```python
from build123d import *

# Parameters (mm, degrees)
F0_R     = 12
F1_DEPTH = 2
F3_DEPTH = 25


with BuildPart() as f1:
    # F0 (on Top) → F1 (new body)
    with BuildSketch(Plane.XY):
        Circle(F0_R)
    extrude(amount=F1_DEPTH)

    # F2 (on face) → F3 (cut)
    with BuildSketch(Plane.XY.offset(2)):
        Polygon((-3.2808869146, 6.2673611111), (-3.2808869146, 7.8645833333), (-5.1267361111, 7.8645833333), (-5.1267361111, -8), (-3.2808869146, -8), (-3.2808869146, -6.4270833333), (-3.2829861111, -6.4270833333), (-3.2829861111, -0.4895833333), (-3.2808869146, -0.4895833333), (-3.2808869146, 1.0729166667), (-3.2829861111, 1.0729166667), (-3.2829861111, 6.2673611111), align=None)
        with BuildLine():
            Line((-0.6440972222, 7.8645833333), (-1.7808869146, 7.8645833333))
            Line((-1.7808869146, 7.8645833333), (-1.7808869146, 6.2673611111))
            Line((-1.7808869146, 6.2673611111), (-0.5677083333, 6.2673611111))
            add(Edge.make_bspline(
                [(2.4704861111, 5.6770833333), (1.515625, 6.2673611111), (-0.5677083333, 6.2673611111)],
                knots=[0, 0, 0, 1, 1, 1], degree=2))
            add(Edge.make_bspline(
                [(3.4253472222, 3.75), (3.4253472222, 5.0868055556), (2.4704861111, 5.6770833333)],
                knots=[0, 0, 0, 1, 1, 1], degree=2))
            add(Edge.make_bspline(
                [(2.5677083333, 1.6857638889), (3.4253472222, 2.2986111111), (3.4253472222, 3.75)],
                knots=[0, 0, 0, 1, 1, 1], degree=2))
            add(Edge.make_bspline(
                [(-0.2447916667, 1.0729166667), (1.7100694444, 1.0729166667), (2.5677083333, 1.6857638889)],
                knots=[0, 0, 0, 1, 1, 1], degree=2))
            Line((-0.2447916667, 1.0729166667), (-1.7808869146, 1.0729166667))
            Line((-1.7808869146, 1.0729166667), (-1.7808869146, -0.4895833333))
            Line((-1.7808869146, -0.4895833333), (-0.1232638889, -0.4895833333))
            add(Edge.make_bspline(
                [(2.8975694444, -1.1840277778), (1.9045138889, -0.4895833333), (-0.1232638889, -0.4895833333)],
                knots=[0, 0, 0, 1, 1, 1], degree=2))
            add(Edge.make_bspline(
                [(3.890625, -3.3541666667), (3.890625, -1.8784722222), (2.8975694444, -1.1840277778)],
                knots=[0, 0, 0, 1, 1, 1], degree=2))
            add(Edge.make_bspline(
                [(2.9201388889, -5.6840277778), (3.890625, -4.9409722222), (3.890625, -3.3541666667)],
                knots=[0, 0, 0, 1, 1, 1], degree=2))
            add(Edge.make_bspline(
                [(0.0295138889, -6.4270833333), (1.9496527778, -6.4270833333), (2.9201388889, -5.6840277778)],
                knots=[0, 0, 0, 1, 1, 1], degree=2))
            Line((0.0295138889, -6.4270833333), (-1.7808869146, -6.4270833333))
            Line((-1.7808869146, -6.4270833333), (-1.7808869146, -8))
            Line((-1.7808869146, -8), (0.4079861111, -8))
            add(Edge.make_bspline(
                [(4.4288194444, -6.8055555556), (2.9913194444, -8), (0.4079861111, -8)],
                knots=[0, 0, 0, 1, 1, 1], degree=2))
            add(Edge.make_bspline(
                [(5.8663194444, -3.4861111111), (5.8663194444, -5.6111111111), (4.4288194444, -6.8055555556)],
                knots=[0, 0, 0, 1, 1, 1], degree=2))
            add(Edge.make_bspline(
                [(2.2517361111, 0.3125), (5.8663194444, -0.3055555556), (5.8663194444, -3.4861111111)],
                knots=[0, 0, 0, 1, 1, 1], degree=2))
            Line((2.2517361111, 0.3125), (2.2517361111, 0.4201388889))
            add(Edge.make_bspline(
                [(4.5486111111, 1.6076388889), (3.7621527778, 0.6909722222), (2.2517361111, 0.4201388889)],
                knots=[0, 0, 0, 1, 1, 1], degree=2))
            add(Edge.make_bspline(
                [(5.3350694444, 3.9375), (5.3350694444, 2.5243055556), (4.5486111111, 1.6076388889)],
                knots=[0, 0, 0, 1, 1, 1], degree=2))
            add(Edge.make_bspline(
                [(3.9236111111, 6.9201388889), (5.3350694444, 5.9756944444), (5.3350694444, 3.9375)],
                knots=[0, 0, 0, 1, 1, 1], degree=2))
            add(Edge.make_bspline(
                [(-0.6440972222, 7.8645833333), (2.5121527778, 7.8645833333), (3.9236111111, 6.9201388889)],
                knots=[0, 0, 0, 1, 1, 1], degree=2))
        make_face()
    extrude(amount=-F3_DEPTH, mode=Mode.SUBTRACT)


solid = f1.part
```
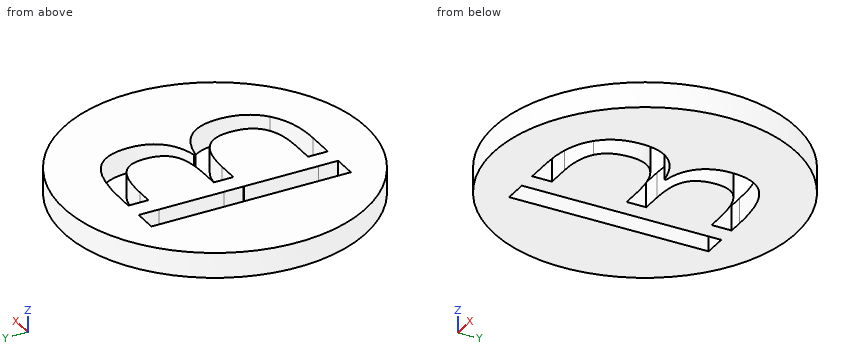
CAD build for the part. Positions are in the model's coordinates, mm. Round coordinates to 2 decimals unless told otherwise and drop trailing zeros. Loops run counter-clockwise (first coordinate to the right, second up) from the corner with the lowest first, then second, coordinate; pieces in that order, holes last. Notation, with made-up numbers: M 22,-13 L 77,-13 A27 cw 77,17 Z; hole C 59.25,41.5 d10. An arc over 180 degrees is marked long. Use a Markdown table: item, result. Add a question column.
(1) Cut at D-D (x = 10.25). Give the cut face in (y, z), and give its area (3 significant figures).
(2) Flat gauge pins, fed straight in: pin 1 (10 mm diameter, centred on x = 2, y = -5.5, fed in from -Z); pin 2 (0.8 mm diameter, centred on y = -7.5, z = 0.5, fed in from +X); pin 3 (0.6 mm diameter, centred on x = -4, z = 1, fed in from -Y); pin 4 (1 mm diameter, centred on y = -4, z = 0.5, fed in from -X). Where does each tip first touch, or does it go through?
(3) Cut at B-B (z = 0.6). State how many separate pieces and enclosed holes the cut face has, and give its area (3 significant figures).
(4) Drill centre lines: line 1 (Y direction, x = 5, z = 0.45); line 2 (X direction, y = -5.5, z = 1.8); line 3 (Y direction, x = -1.5, z = 0.6). Where is each one in solid material? Low to high.
(5) Cut at A-A (x = -4.75). Give the cut face in (y, z), and give its area (3 significant figures).
Geometry says:
| question | item | result |
|---|---|---|
| 1 | outline | M -6.24,0 L 6.24,0 L 6.24,2 L -6.24,2 Z |
| 1 | area | 25.0 mm² |
| 2 | pin 1 | stops at z = 0 |
| 2 | pin 2 | stops at x = 9.67 |
| 2 | pin 3 | stops at y = -11.42 |
| 2 | pin 4 | stops at x = -11.48 |
| 3 | separate pieces | 1 |
| 3 | enclosed holes | 2 |
| 3 | area | 374 mm² |
| 4 | line 1 | y = -10.91 to -6.22, -0.99 to 2.3, 5.66 to 10.91 |
| 4 | line 2 | x = -10.67 to -5.13, -3.28 to 3.13, 5.45 to 10.67 |
| 4 | line 3 | y = -11.91 to -8, -6.43 to -0.49, 1.07 to 6.27, 7.86 to 11.91 |
| 5 | outline | M -11.02,0 L -8,0 L -8,2 L -11.02,2 Z; M 7.86,0 L 11.02,0 L 11.02,2 L 7.86,2 Z |
| 5 | area | 12.4 mm² |
